Geometry check sheet. Reference: the model listing, model coordinates, mm. A direction names the side the tool comes from. Round coordinates to 2 decimals unless told otherwise and drop trailing zeros. Order: outer loops, then holes, each group sorted by start corner. A loop starts at its lowest first (then second) coordinate and runs counter-clockwise, first axis right, second up. Notation, with made-up numbers: M 77.5,68.25 L 91.5,68.25 A17 ccw 91.5,78.25 Z; hole C 51,26.5 d11. An arc over 180 degrees is marked long. Return JSON: item names as keys, results as strings. Group by question number.
```python
from build123d import *

# Parameters (mm, degrees)
BOSS_EXTRUDE1_DEPTH        = 2.5
F_12_0MM_DOWEL_HOLE1_D     = 12
F_12_0MM_DOWEL_HOLE1_DEPTH = 5
F_8_0MM_DOWEL_HOLE1_D      = 8.2
F_8_0MM_DOWEL_HOLE1_DEPTH  = 5


with BuildPart() as part:
    # Sketch1 → Boss-Extrude1 (new body, symmetric)
    with BuildSketch(Plane(origin=(0, 0, 0), x_dir=(1, 0, 0), z_dir=(0, 1, 0))):
        with BuildLine():
            Line((-88.9, 30), (-127, 30))
            ThreePointArc((-127, 30), (-157, 0), (-127, -30))
            Line((-127, -30), (-88.9, -30))
            ThreePointArc((-88.9, -30), (-76.2, -42.7), (-63.5, -30))
            Line((-63.5, -30), (127, -30))
            ThreePointArc((127, -30), (157, 0), (127, 30))
            Line((127, 30), (-63.5, 30))
            ThreePointArc((-63.5, 30), (-76.2, 42.7), (-88.9, 30))
        make_face()
    extrude(amount=BOSS_EXTRUDE1_DEPTH, both=True)

    # Ø12.0mm Dowel Hole1
    with Locations(Plane(origin=(0, 2.5, 0), x_dir=(1, 0, 0), z_dir=(0, 1, 0))):
        with Locations((-127, 0), (127, 0)):
            Hole(F_12_0MM_DOWEL_HOLE1_D / 2, depth=F_12_0MM_DOWEL_HOLE1_DEPTH)

    # Ø8.0mm Dowel Hole1
    with Locations(Plane(origin=(0, 2.5, 0), x_dir=(1, 0, 0), z_dir=(0, 1, 0))):
        with Locations((-76.2, 30), (-76.2, -30)):
            Hole(F_8_0MM_DOWEL_HOLE1_D / 2, depth=F_8_0MM_DOWEL_HOLE1_DEPTH)


solid = part.part
```
Q1. Section check B-B on y = 1.5. Record the cut outline in (x, z).
Q2. Section check D-D on x = 138. Record the cut outline in (y, z), plus the area to 3 significant figures.
Q3. Section check A-A on x = -76.2. Record the cut outline in (y, z).
Q4. Section check C-C on z = 18. Record the cut outline in (x, y), plus the area to 3 significant figures.
Q5. Set-up check for faces 1 (the face through (-108, 0, -30)), 2 (the face through (33, 0, -30)), 3 (the face through (-108, 0, 30)): record each of +Z, -Z, +X, -X, +Y, -Y from which the full face is reachable in a straight line by a thin tool's end or side.
Q6. Release check for a two-part mould opening along Z. For faces 4 (the face through (-2, -2.5, -1)), 5 (the face through (156.993, 0.035, 0.66)), 6 (the face through (131.76, -0.04, 3.65)) record: +Z half, -Z half, draft (parallel to the pull), parting line (faces both ways), or undercut.
Q7. Depth check by flat-ended pin: pin 1 Ø1.5 at (x, y) = (-109, -0.5) entering from -Z; pin 2 Ø1.5 at (x, y) = (2, 1) entering from +Z; pin 3 Ø5 at (x, z) = (-76.2, 30) entering from +Y. Enter the tip coordinate at first touch or a pass-through.
Q8. Material ranges on line 1 along Z through (x, y) = (-76.2, 0.5); line 2 along Z through (x, y) = (-62.5, 1.8); line 3 along Z through (x, y) = (-127, -1.3), recorded low to high.
Geometry check:
{
 "1": {"outline": "M -127,-30 L -88.9,-30 A12.7 ccw -63.5,-30 L 127,-30 A30 ccw 127,30 L -63.5,30 A12.7 ccw -88.9,30 L -127,30 A30 ccw Z; hole C -127,0 d12; hole C -76.2,-30 d8.2; hole C -76.2,30 d8.2; hole C 127,0 d12"},
 "2": {"outline": "M -2.5,-27.91 L 2.5,-27.91 L 2.5,27.91 L -2.5,27.91 Z", "area": "279 mm^2"},
 "3": {"outline": "M -2.5,-42.7 L 2.5,-42.7 L 2.5,-34.1 L -2.5,-34.1 Z; M -2.5,-25.9 L 2.5,-25.9 L 2.5,25.9 L -2.5,25.9 Z; M -2.5,34.1 L 2.5,34.1 L 2.5,42.7 L -2.5,42.7 Z"},
 "4": {"outline": "M -151,-2.5 L 151,-2.5 L 151,2.5 L -151,2.5 Z", "area": "1,510 mm^2"},
 "5": {"face 1": "-Z, -X, +Y, -Y", "face 2": "-Z, +X, +Y, -Y", "face 3": "+Z, -X, +Y, -Y"},
 "6": {"face 4": "draft", "face 5": "parting line", "face 6": "undercut"},
 "7": {"pin 1": "stops at z = -30", "pin 2": "stops at z = 30", "pin 3": "passes through"},
 "8": {"line 1": "z = -42.7 to -34.1, -25.9 to 25.9, 34.1 to 42.7", "line 2": "z = -30 to 30", "line 3": "z = -30 to -6, 6 to 30"}
}
